Could you check a few things on this model? Use its own coordinates, in mm. Face numbers are marked on the shaded views. A direction names the side the tool comes from. Give positions to 0.01 mm unless a question says otherwise; leave off trailing zeros. Order: outer loops, then holes, each group sorted by start corner. A loop starts at its lowest first (then second) coordinate and runs counter-clockwise, first axis right, second up.
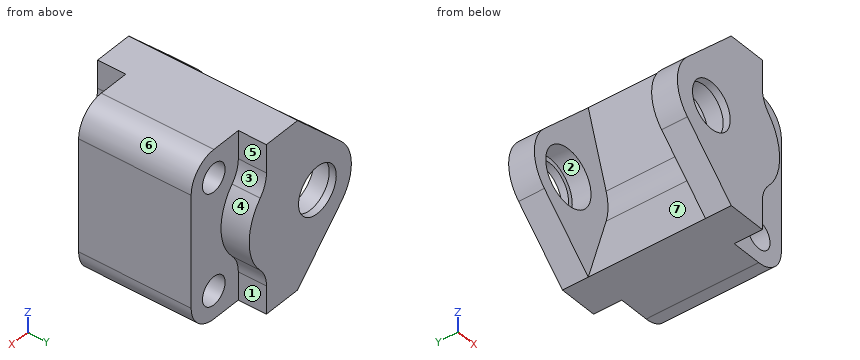
from build123d import *

# Parameters (mm, degrees)
SKETCH1_R           = 1.5
BOSS_EXTRUDE1_DEPTH = 9
CUT_EXTRUDE1_DEPTH  = 6.25
CUT_EXTRUDE2_START  = 9
CUT_EXTRUDE2_DEPTH  = 3
CUT_EXTRUDE3_START  = -6
CUT_EXTRUDE3_DEPTH  = 3


with BuildPart() as part:
    # Sketch1 → Boss-Extrude1 (new, symmetric)
    with BuildSketch(Plane(origin=(0, 0, 0), x_dir=(1, 0, 0), z_dir=(0, 1, 0))):
        with BuildLine():
            Line((13, 6), (13, -6))
            ThreePointArc((13, -6), (12.121320344, -8.121320344), (10, -9))
            Line((10, -9), (2.636038969, -9))
            Line((2.636038969, -9), (-3.181980515, -3.181980515))
            ThreePointArc((-3.181980515, -3.181980515), (-4.5, 0), (-3.181980515, 3.181980515))
            Line((-3.181980515, 3.181980515), (2.636038969, 9))
            Line((2.636038969, 9), (10, 9))
            ThreePointArc((10, 9), (12.121320344, 8.121320344), (13, 6))
        make_face()
        with Locations(Location((10, 6, 0), (0, 0, 270))):
            Circle(SKETCH1_R, mode=Mode.SUBTRACT)
        with Locations(Location((10, -6, 0), (0, 0, 270))):
            Circle(SKETCH1_R, mode=Mode.SUBTRACT)
    extrude(amount=BOSS_EXTRUDE1_DEPTH, both=True)

    # Sketch2 → Cut-Extrude1 (cut, symmetric)
    with BuildSketch(Plane(origin=(0, 0, 0), x_dir=(1, 0, 0), z_dir=(0, 1, 0))):
        with BuildLine():
            Line((5.000969408, 1.597749973), (2.636038969, 9))
            Line((2.636038969, 9), (-3.181980515, 3.181980515))
            ThreePointArc((-3.181980515, 3.181980515), (-4.5, 0), (-3.181980515, -3.181980515))
            Line((-3.181980515, -3.181980515), (2.636038969, -9))
            Line((2.636038969, -9), (5.000969408, -1.597749973))
            ThreePointArc((5.000969408, -1.597749973), (5.25, 0), (5.000969408, 1.597749973))
        make_face()
    extrude(amount=CUT_EXTRUDE1_DEPTH, both=True, mode=Mode.SUBTRACT)

    # Sketch3 → Cut-Revolve1 (revolve, cut)
    with BuildSketch(Plane.XY, mode=Mode.PRIVATE) as cut_revolve1_sk:
        Polygon((-2.5, 9), (-2.5, 8.25), (-3, 8.25), (-3, 6.25), (0, 6.25), (0, 9), align=None)
        Polygon((0, -6.25), (0, -9), (-2.5, -9), (-2.5, -8.25), (-3, -8.25), (-3, -6.25), align=None)
    revolve(cut_revolve1_sk.sketch.rotate(Axis((0, -11.503843925, 0), (0, 1, 0)), 270), axis=Axis((0, -11.503843925, 0), (0, 1, 0)), mode=Mode.SUBTRACT)

    # Sketch4 → Cut-Extrude2 (cut)
    with BuildSketch(Plane(origin=(0, 0, 0), x_dir=(1, 0, 0), z_dir=(0, 1, 0)).offset(CUT_EXTRUDE2_START)):
        with BuildLine():
            Line((6.75, -9), (10, -9))
            ThreePointArc((10, -9), (12.121320344, -8.121320344), (13, -6))
            Line((13, -6), (13, 6))
            ThreePointArc((13, 6), (12.121320344, 8.121320344), (10, 9))
            Line((10, 9), (6.75, 9))
            Line((6.75, 9), (6.75, 6))
            ThreePointArc((6.75, 6), (6.963939833, 4.840328208), (7.577593024, 3.833333333))
            ThreePointArc((7.577593024, 3.833333333), (9.041796068, 0), (7.577593024, -3.833333333))
            ThreePointArc((7.577593024, -3.833333333), (6.963939833, -4.840328208), (6.75, -6))
            Line((6.75, -6), (6.75, -9))
        make_face()
    extrude(amount=-CUT_EXTRUDE2_DEPTH, mode=Mode.SUBTRACT)

    # Sketch4<2> → Cut-Extrude3 (cut)
    with BuildSketch(Plane(origin=(0, 0, 0), x_dir=(1, 0, 0), z_dir=(0, 1, 0)).offset(CUT_EXTRUDE3_START)):
        with BuildLine():
            Line((6.75, -9), (10, -9))
            ThreePointArc((10, -9), (12.121320344, -8.121320344), (13, -6))
            Line((13, -6), (13, 6))
            ThreePointArc((13, 6), (12.121320344, 8.121320344), (10, 9))
            Line((10, 9), (6.75, 9))
            Line((6.75, 9), (6.75, 6))
            ThreePointArc((6.75, 6), (6.963939833, 4.840328208), (7.577593024, 3.833333333))
            ThreePointArc((7.577593024, 3.833333333), (9.041796068, 0), (7.577593024, -3.833333333))
            ThreePointArc((7.577593024, -3.833333333), (6.963939833, -4.840328208), (6.75, -6))
            Line((6.75, -6), (6.75, -9))
        make_face()
    extrude(amount=-CUT_EXTRUDE3_DEPTH, mode=Mode.SUBTRACT)


solid = part.part
Item 1: We'd pull the mould along Z, two halves only. Please class the marked faces 5, 6 and 7: +Z half, -Z half, draft (parallel to the pull), parting line (faces both ways), or undercut.
Findings:
face 5: draft
face 6: +Z half
face 7: undercut
Item 2: For the marked faces 1, 2, 3 and 4, which set-ups out of +Z, -Z, +X, -X, +Y, -Y let a thin tool reach every point of the face, with its end or its side?
Findings:
face 1: -Z, +X, +Y
face 2: none
face 3: +Z, +X, +Y
face 4: +X, +Y
Item 3: Imagine slicing it at B-B on z = 0. List the corners of the cut face in (x, y) for me.
Findings:
outline: (-4.5, -9) - (-2.5, -9) - (-2.5, -8.25) - (-3, -8.25) - (-3, -6.25) - (-4.5, -6.25) - close; (-4.5, 6.25) - (-3, 6.25) - (-3, 8.25) - (-2.5, 8.25) - (-2.5, 9) - (-4.5, 9) - close; (2.5, -9) - (9.04, -9) - (9.04, -6) - (13, -6) - (13, 6) - (9.04, 6) - (9.04, 9) - (2.5, 9) - (2.5, 8.25) - (3, 8.25) - (3, 6.25) - (5.25, 6.25) - (5.25, -6.25) - (3, -6.25) - (3, -8.25) - (2.5, -8.25) - close
Item 4: Imagine slicing it at C-C on x = 3.5. List the corners of the cut face in (y, z) for me.
Findings:
outline: (-9, -9) - (9, -9) - (9, 9) - (-9, 9) - close; hole (-6.25, -6.3) - (6.25, -6.3) - (6.25, 6.3) - (-6.25, 6.3) - close
Item 5: Imagine slicing it at A-A on y = 1. List the corners of the cut face in (x, z) for me, then the cut area to 3 significant figures.
Findings:
outline: (2.64, -9) - (10, -9) arc R3 ccw to (13, -6) - (13, 6) arc R3 ccw to (10, 9) - (2.64, 9) - (5, 1.6) arc R5.25 cw to (5, -1.6) - close; hole circle Ø3 at (10, -6); hole circle Ø3 at (10, 6)
area: 143 mm2
Item 6: Please list where these lines run through material, in increasing order: line 1 along Z through (x, y) = (10, 1); line 2 along X through (y, z) = (-7.35, 0); line 3 along Y through (x, z) = (1.25, -6).
Findings:
line 1: z = -9 to -7.5, -4.5 to 4.5, 7.5 to 9
line 2: x = -4.5 to -3, 3 to 9.04
line 3: y = -9 to -6.25, 6.25 to 9
Item 7: Imagine slicing it at D-D on x = -1.75. List the corners of the cut face in (y, z) for me.
Findings:
outline: (-9, -4.61) - (-6.25, -4.61) - (-6.25, -2.44) - (-8.25, -2.44) - (-8.25, -1.79) - (-9, -1.79) - close; (-9, 1.79) - (-8.25, 1.79) - (-8.25, 2.44) - (-6.25, 2.44) - (-6.25, 4.61) - (-9, 4.61) - close; (6.25, -4.61) - (9, -4.61) - (9, -1.79) - (8.25, -1.79) - (8.25, -2.44) - (6.25, -2.44) - close; (6.25, 2.44) - (8.25, 2.44) - (8.25, 1.79) - (9, 1.79) - (9, 4.61) - (6.25, 4.61) - close
Item 8: For pin 1 (3 mm diameter, centred on x = 11.5, z = -3.5, fed in from -Y); pin 2 (5 mm diameter, centred on x = -0.5, y = -6.5, fed in from -Z); pin 3 (1.5 mm diameter, centred on y = 8, z = -7.5, fed in from +X), each with a flat end and sliding along its axis, tell me the tip position at first contact or that it passes through.
Findings:
pin 1: stops at y = -6
pin 2: stops at z = -8.36
pin 3: stops at x = 6.75
